Build history of the part. All positions in model axes, mm. A direction names the side the tool comes from. Give positions to 0.01 mm unless a question says otherwise; leave off trailing zeros. Write each loop counter-clockwise with the first axis right and the second up, starting at its lowest first coordinate (ties: lowest second). Pieces come first, ordered by that corner, then holes. Notation, with made-up numbers: (31, 44.5) -> (39, 44.5) arc R19 cw to (39, 56.5) -> close; hole circle Ø6 at (41.25, 14). An arc over 180 degrees is marked (long way). One line per question, with ' | ' between items. Start each with the question number.
(1) Band-saw the part on C-C, the plane y = 17. Give the cut face in (x, z), and give its area (3 significant figures).
(2) Drill centre lines: probe 1 along Y at (x, z) = (-24.45, 0); probe 2 along Y at (x, z) = (-24.2, 15.5); probe 3 along Y at (x, z) = (23.75, -17.5). Where is each one in solid material? Low to high. Write a range as from..to.
(3) Band-saw the part on A-A, the plane z = 15.5. Give the cut face in (x, y), and give its area (3 significant figures).
(4) Band-saw the part on B-B, the plane z = 0. Count the separate pieces of the cut face and the enclosed holes in it, and give its area (3 significant figures).
(5) Pin check, flat tips, straight feed: P1, Ø5, axis at x = -1.5, z = 4, coming from the +Y side; P2, Ø2.5, axis at y = 6.5, z = 15.5, coming from the +X side. Stop position of each tip, or through.
(6) Tool access for faces 1 (the cylindrical face through (23.73, 36.53, -16.77)), 2 (the flat face through (22, 31, 10)): list every direction of +Z, -Z, +X, -X, +Y, -Y with a clear straight run to the whole face (end or side of a thin tool).
(7) Pull direction X, two halves, no side cores. Call faces 3 (the flat face through (0, 0, 0)), 4 (the flat face through (-22, 31, 10)), 5 (the flat face through (-25.5, 10, 0)), 6 (the flat face through (24, 44, 0)): released by +X, released by -X, zero draft, split by the parting line, or undercut.
(8) Band-saw the part on D-D, the plane x = 1. Give the cut face in (y, z).
from build123d import *

# Parameters (mm, degrees)
SKETCH1_W                     = 44
SKETCH1_H                     = 44
BOSS_EXTRUDE1_DEPTH           = 3.5
SKETCH3_W                     = 3.5
SKETCH3_H                     = 44
BOSS_EXTRUDE2_DEPTH           = 44
BOSS_EXTRUDE2_DEPTH_BACK      = 3.5
SKETCH4_W                     = 3.5
SKETCH4_H                     = 44
BOSS_EXTRUDE3_DEPTH           = 44
BOSS_EXTRUDE3_DEPTH_BACK      = 3.5
SKETCH5_R                     = 11.25
CUT_EXTRUDE1_DEPTH            = 26.5
CUT_EXTRUDE1_DEPTH_BACK       = 26.5
M3_CLEARANCE_HOLE1_D          = 3.2
SKETCH16_W                    = 1.6
SKETCH16_H                    = 25.5
M3_CLEARANCE_HOLE2_AT_2_COUNT = 2
M3_CLEARANCE_HOLE2_AT_2_PITCH = 24.748737342
M3_CLEARANCE_HOLE2_AT_3_COUNT = 2
M3_CLEARANCE_HOLE2_AT_3_PITCH = 24.748737342
M3_CLEARANCE_HOLE3_D          = 3.2


with BuildPart() as part:
    # Sketch1 → Boss-Extrude1 (new body)
    with BuildSketch(Plane(origin=(0, 0, 0), x_dir=(1, 0, 0), z_dir=(0, 1, 0))):
        Rectangle(SKETCH1_W, SKETCH1_H)
    extrude(amount=-BOSS_EXTRUDE1_DEPTH)

    # Sketch3 → Boss-Extrude2 (add, two sides)
    with BuildSketch(Plane(origin=(0, 0, 0), x_dir=(1, 0, 0), z_dir=(0, 1, 0))) as boss_extrude2_sk:
        with Locations((23.75, 0)):
            Rectangle(SKETCH3_W, SKETCH3_H)
    extrude(amount=BOSS_EXTRUDE2_DEPTH)
    extrude(boss_extrude2_sk.sketch, amount=-BOSS_EXTRUDE2_DEPTH_BACK)

    # Sketch4 → Boss-Extrude3 (add, two sides)
    with BuildSketch(Plane(origin=(0, 0, 0), x_dir=(1, 0, 0), z_dir=(0, 1, 0))) as boss_extrude3_sk:
        with Locations((-23.75, 0)):
            Rectangle(SKETCH4_W, SKETCH4_H)
    extrude(amount=BOSS_EXTRUDE3_DEPTH)
    extrude(boss_extrude3_sk.sketch, amount=-BOSS_EXTRUDE3_DEPTH_BACK)

    # Sketch5 → Cut-Extrude1 (cut, two sides)
    with BuildSketch(Plane(origin=(0, 0, 0), x_dir=(0, 0, -1), z_dir=(1, 0, 0))) as cut_extrude1_sk:
        with Locations((0, 22)):
            Circle(SKETCH5_R)
    extrude(amount=CUT_EXTRUDE1_DEPTH, mode=Mode.SUBTRACT)
    extrude(cut_extrude1_sk.sketch, amount=-CUT_EXTRUDE1_DEPTH_BACK, mode=Mode.SUBTRACT)

    # M3 Clearance Hole1 (through all)
    with Locations(Plane(origin=(25.5, 0, 0), x_dir=(0, 0, -1), z_dir=(1, 0, 0))):
        with Locations((-15.5, 6.5), (-15.5, 37.5), (15.5, 37.5), (15.5, 6.5)):
            Hole(M3_CLEARANCE_HOLE1_D / 2)

    # Sketch16 → M3 Clearance Hole2 (revolve, cut)
    with BuildSketch(Plane(origin=(0, 22, -17.5), x_dir=(0, 0, 1), z_dir=(0, 1, 0))):
        with Locations((0.8, 12.75)):
            Rectangle(SKETCH16_W, SKETCH16_H)
    m3_clearance_hole2 = revolve(axis=Axis((-6.35, 22, -17.5), (1, 0, 0)), mode=Mode.SUBTRACT)

    # M3 Clearance Hole2 at 2: M3 Clearance Hole2 ×2
    with Locations(*[Vector(0, 0.707106781, 0.707106781) * (i * M3_CLEARANCE_HOLE2_AT_2_PITCH) for i in range(1, M3_CLEARANCE_HOLE2_AT_2_COUNT)]):
        add(m3_clearance_hole2, mode=Mode.SUBTRACT)

    # M3 Clearance Hole2 at 3: M3 Clearance Hole2 ×2
    with Locations(*[Vector(0, -0.707106781, 0.707106781) * (i * M3_CLEARANCE_HOLE2_AT_3_PITCH) for i in range(1, M3_CLEARANCE_HOLE2_AT_3_COUNT)]):
        add(m3_clearance_hole2, mode=Mode.SUBTRACT)

    # M3 Clearance Hole3 (through all)
    with Locations(Plane.ZY.offset(25.5)):
        with Locations((0, 4.5), (0, 39.5), (-17.5, 22)):
            Hole(M3_CLEARANCE_HOLE3_D / 2)


solid = part.part
Results:
1) outline: (-25.5, -22) -> (-22, -22) -> (-22, -10.08) -> (-25.5, -10.08) -> close; (-25.5, 10.08) -> (-22, 10.08) -> (-22, 22) -> (-25.5, 22) -> close; (22, -22) -> (25.5, -22) -> (25.5, -10.08) -> (22, -10.08) -> close; (22, 10.08) -> (25.5, 10.08) -> (25.5, 22) -> (22, 22) -> close | area: 167 mm²
2) probe 1: y = -3.5..2.9, 6.1..10.75, 33.25..37.9, 41.1..44 | probe 2: y = -3.5..4.9, 8.1..35.9, 39.1..44 | probe 3: y = -3.5..20.4, 23.6..44
3) outline: (-25.5, -3.5) -> (25.5, -3.5) -> (25.5, 4.9) -> (22, 4.9) -> (22, 0) -> (-22, 0) -> (-22, 4.9) -> (-25.5, 4.9) -> close; (-25.5, 8.1) -> (-22, 8.1) -> (-22, 35.9) -> (-25.5, 35.9) -> close; (-25.5, 39.1) -> (-22, 39.1) -> (-22, 44) -> (-25.5, 44) -> close; (22, 8.1) -> (25.5, 8.1) -> (25.5, 35.9) -> (22, 35.9) -> close; (22, 39.1) -> (25.5, 39.1) -> (25.5, 44) -> (22, 44) -> close | area: 442 mm²
4) separate pieces: 7 | enclosed holes: 0 | area: 284 mm²
5) P1: stops at y = 0 | P2: passes through
6) face 1: +X, -X | face 2: +Z, -Z, +Y
7) face 3: undercut | face 4: undercut | face 5: released by -X | face 6: zero draft
8) outline: (-3.5, -22) -> (0, -22) -> (0, 22) -> (-3.5, 22) -> close
